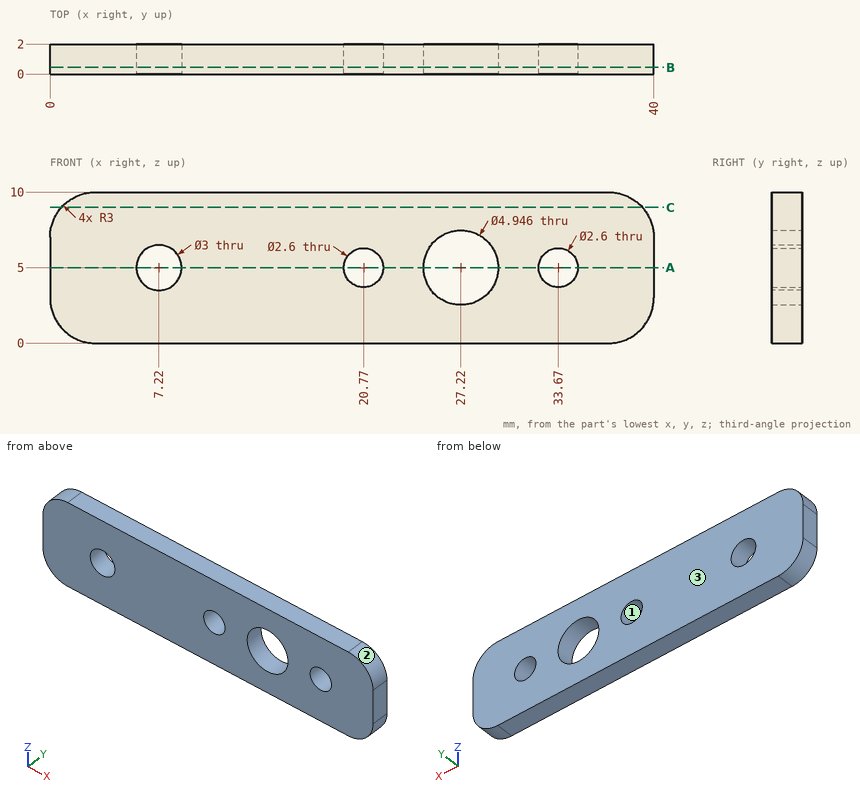
Here's the drawing with two shaded views (mm, measured from the low corner). I have some questions. Give positions to 0.01 mm unless a question says otherwise; leave off trailing zeros. Order: outer loops, then holes, each group sorted by start corner. A loop starts at its lowest first (then second) coordinate and runs counter-clockwise, first axis right, second up.
Q1. Suppose I cut it at B-B, the plane y = 0.45. Write out the boundary of the cut face in (x, z).
Q2. I'm going to push flat-ended pins straight in: P1, Ø1, axis at x = 31.5, y = 1.5, coming from the -Z side; P2, Ø4, axis at x = 27.22, z = 5, coming from the -Y side. Where does each tip first touch, or does it pass through?
Q3. We'd pull the mould along Z, two halves only. Please class the marked faces 1, 2 and 3: +Z half, -Z half, draft (parallel to the pull), parting line (faces both ways), or undercut.
Q4. Suppose I cut it at C-C, the plane z = 9. Write out the boundary of the cut face in (x, y).
Q5. Suppose I cut it at A-A, the plane z = 5. Write out the boundary of the cut face in (x, y), and give its area (3 significant figures).
Q6. If I drill on line 1 along X through (y, z) = (1.6, 5); line 2 along X through (y, z) = (1.65, 5.75) (1 decimal); line 3 along X through (y, z) = (0.3, 7) (1 decimal), over which ranges is the centre line in solid material (lowest first)?
Solution:
1. outline: (0, 3) arc R3 ccw to (3, 0) - (37, 0) arc R3 ccw to (40, 3) - (40, 7) arc R3 ccw to (37, 10) - (3, 10) arc R3 ccw to (0, 7) - close; hole circle Ø3 at (7.22, 5); hole circle Ø2.6 at (20.77, 5); hole circle Ø4.95 at (27.22, 5); hole circle Ø2.6 at (33.67, 5)
2. P1: stops at z = 0
2. P2: passes through
3. face 1: undercut
3. face 2: +Z half
3. face 3: draft
4. outline: (0.76, 0) - (39.24, 0) - (39.24, 2) - (0.76, 2) - close
5. outline: (0, 0) - (5.72, 0) - (5.72, 2) - (0, 2) - close; (8.72, 0) - (19.47, 0) - (19.47, 2) - (8.72, 2) - close; (22.07, 0) - (24.75, 0) - (24.75, 2) - (22.07, 2) - close; (29.69, 0) - (32.37, 0) - (32.37, 2) - (29.69, 2) - close; (34.97, 0) - (40, 0) - (40, 2) - (34.97, 2) - close
5. area: 53.7 mm2
6. line 1: x = 0 to 5.72, 8.72 to 19.47, 22.07 to 24.75, 29.69 to 32.37, 34.97 to 40
6. line 2: x = 0 to 5.9, 8.5 to 19.7, 21.8 to 24.9, 29.6 to 32.6, 34.7 to 40
6. line 3: x = 0 to 25.8, 28.7 to 40
